The listing builds one solid part. Answer for the finished solid, in the listing's coordinates (mm). Face numbers are marked on the shaded views. A direction names the side the tool comes from. Round coordinates to 2 decimals unless told otherwise and drop trailing zeros. Write each loop counter-clockwise with the first axis right and the second up, starting at its lowest first coordinate (ties: lowest second). Pieces come first, ordered by that corner, then holes.
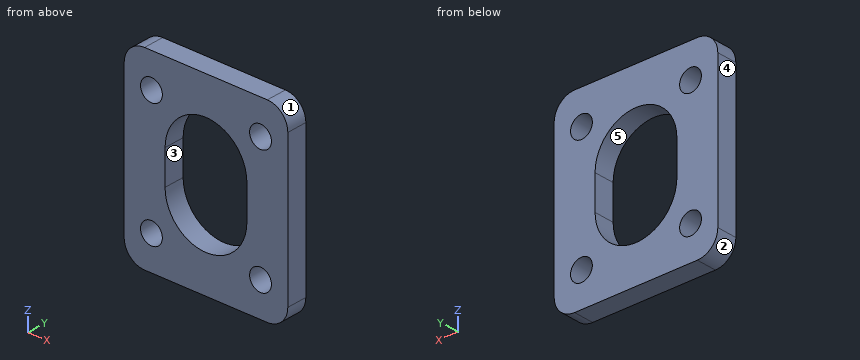
from build123d import *

# Parameters (mm, degrees)
SKETCH_1_W      = 24
SKETCH_1_H      = 28
SKETCH_1_R      = 1.6
EXTRUDE_1_DEPTH = 3
FILLET_1_R      = 3


with BuildPart() as part:
    # 草图1 → 凸台-拉伸1 (new body)
    with BuildSketch(Plane(origin=(0, 0, 0), x_dir=(1, 0, 0), z_dir=(0, 1, 0))):
        Rectangle(SKETCH_1_W, SKETCH_1_H)
        with Locations(Location((8, -9, 0), (0, 0, 270))):
            Circle(SKETCH_1_R, mode=Mode.SUBTRACT)
        with Locations(Location((-8, -9, 0), (0, 0, 270))):
            Circle(SKETCH_1_R, mode=Mode.SUBTRACT)
        with Locations(Location((-8, 9, 0), (0, 0, 270))):
            Circle(SKETCH_1_R, mode=Mode.SUBTRACT)
        with Locations(Location((8, 9, 0), (0, 0, 270))):
            Circle(SKETCH_1_R, mode=Mode.SUBTRACT)
        with BuildLine():
            Line((6, 2.5), (6, -2.5))
            ThreePointArc((6, -2.5), (0, -8.5), (-6, -2.5))
            Line((-6, -2.5), (-6, 2.5))
            ThreePointArc((-6, 2.5), (0, 8.5), (6, 2.5))
        make_face(mode=Mode.SUBTRACT)
    extrude(amount=EXTRUDE_1_DEPTH)

    # 圆角1
    fillet_1_edges = [part.edges().sort_by_distance(p)[0] for p in [
        (12, 1.5, 14),
        (-12, 1.5, 14),
        (-12, 1.5, -14),
        (12, 1.5, -14),
    ]]
    fillet(fillet_1_edges, radius=FILLET_1_R)


solid = part.part
1. Straight lines are drawn through the part: line 1 along X through (y, z) = (0.9, -9); line 2 along X through (y, z) = (0.4, -1.5); line 3 along Z through (x, y) = (-9.25, 2.25). For each, find the intervals that lie inside material, in ascending order.
Geometry says:
line 1: x = -12 to -9.6, -6.4 to 6.4, 9.6 to 12
line 2: x = -12 to -6, 6 to 12
line 3: z = -13.99 to -10, -8 to 8, 10 to 13.99
2. A tool of negligible diameter and unlimited length cuts with its end or side. For the marked faces 4 and 5, from which of +Z, -Z, +X, -X, +Y, -Y can it reach the whole face along a straight path? Write none if from no direction.
Geometry says:
face 4: +Z, -Z, -X, +Y, -Y
face 5: +Y, -Y
3. Section C-C on y = 2.65 is taken. Determine the outline of the cut face in (x, z).
Geometry says:
outline: (-12, -11) arc R3 ccw to (-9, -14) - (9, -14) arc R3 ccw to (12, -11) - (12, 11) arc R3 ccw to (9, 14) - (-9, 14) arc R3 ccw to (-12, 11) - close; hole circle Ø3.2 at (-8, -9); hole circle Ø3.2 at (-8, 9); hole (-6, -2.5) arc R6 ccw to (6, -2.5) - (6, 2.5) arc R6 ccw to (-6, 2.5) - close; hole circle Ø3.2 at (8, -9); hole circle Ø3.2 at (8, 9)
4. Section A-A on x = 0 is taken. Determine the outline of the cut face in (y, z), plus the area to 3 significant figures.
Geometry says:
outline: (0, -14) - (3, -14) - (3, -8.5) - (0, -8.5) - close; (0, 8.5) - (3, 8.5) - (3, 14) - (0, 14) - close
area: 33.0 mm2
5. Given pin 1 (2.5 mm diameter, centred on x = 8, z = 9, fed in from +Y), flat-ended and moving along its own axis, determine where the tip first touches the part or whether it passes through.
Geometry says:
pin 1: passes through
6. For a pull along Z with two mould halves and no side action, classify the marked faces 1, 2 and 3 as released by +Z, released by -Z, zero draft, split by the parting line, or undercut.
Geometry says:
face 1: released by +Z
face 2: released by -Z
face 3: undercut
7. Section D-D on z = -9.75 is taken. Determine the outline of the cut face in (x, y), plus the area to 3 significant figures.
Geometry says:
outline: (-12, 0) - (-9.41, 0) - (-9.41, 3) - (-12, 3) - close; (-6.59, 0) - (6.59, 0) - (6.59, 3) - (-6.59, 3) - close; (9.41, 0) - (12, 0) - (12, 3) - (9.41, 3) - close
area: 55.0 mm2
8. Section B-B on x = -8 is taken. Determine the outline of the cut face in (y, z).
Geometry says:
outline: (0, -14) - (3, -14) - (3, -10.6) - (0, -10.6) - close; (0, -7.4) - (3, -7.4) - (3, 7.4) - (0, 7.4) - close; (0, 10.6) - (3, 10.6) - (3, 14) - (0, 14) - close
